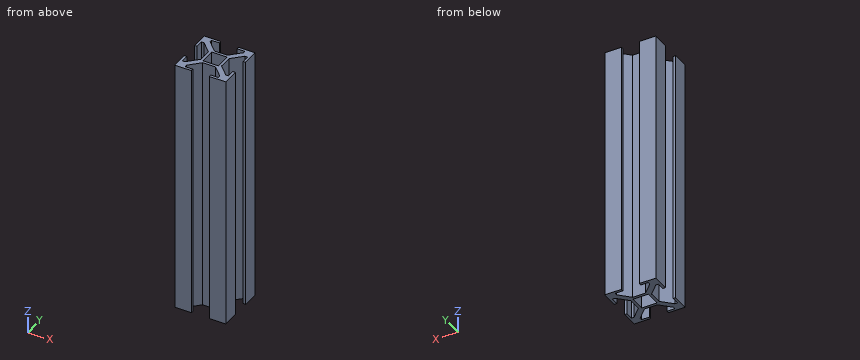
from build123d import *

# Parameters (mm, degrees)
SKETCH_W        = 20
SKETCH_H        = 20
PAD_DEPTH       = 100
SKETCH001_W     = 6
SKETCH001_H     = 6
POCKET_DEPTH    = 100.001
POCKET001_DEPTH = 100.001


with BuildPart() as part:
    # Sketch → Pad (new body)
    with BuildSketch(Plane.XY):
        with Locations((10, 10)):
            Rectangle(SKETCH_W, SKETCH_H)
    extrude(amount=PAD_DEPTH)

    # Sketch001 (on Face6 of Pad) → Pocket (cut, through all)
    with BuildSketch(Plane.XY.offset(100)):
        with Locations((10, 10)):
            Rectangle(SKETCH001_W, SKETCH001_H)
    extrude(amount=-POCKET_DEPTH, mode=Mode.SUBTRACT)

    # Sketch002 (on Face5 of Pocket) → Pocket001 (cut, through all)
    with BuildSketch(Plane.XY.offset(100)):
        Polygon((0, 6.5), (1, 6.5), (1, 3.5), (2, 3.5), (6, 7.5), (6, 12.5), (2, 16.5), (1, 16.5), (1, 13.5), (0, 13.5), align=None)
        Polygon((6.5, 0), (6.5, 1), (3.5, 1), (3.5, 2), (7.5, 6), (12.5, 6), (16.5, 2), (16.5, 1), (13.5, 1), (13.5, 0), align=None)
        Polygon((20, 6.5), (19, 6.5), (19, 3.5), (18, 3.5), (14, 7.5), (14, 12.5), (18, 16.5), (19, 16.5), (19, 13.5), (20, 13.5), align=None)
        Polygon((6.5, 20), (6.5, 19), (3.5, 19), (3.5, 18), (7.5, 14), (12.5, 14), (16.5, 18), (16.5, 19), (13.5, 19), (13.5, 20), align=None)
    extrude(amount=-POCKET001_DEPTH, mode=Mode.SUBTRACT)


solid = part.part
Can you work these out from the model? Positions are in its coordinate system, mm. Give positions to 0.01 mm unless a question says otherwise; leave off trailing zeros. Loops run counter-clockwise (first coordinate to the right, second up) from the corner with the lowest first, then second, coordinate; pieces in that order, holes last. Notation, with made-up numbers: M -17,-8.5 L -7,-8.5 A12 cw -7,-2.5 Z; hole C 26.5,-6 d4. An arc over 180 degrees is marked long. One line per item, written item: value. Start each with the question number.
1) If we section it at A-A, the plane y = 10.5: Write out the boundary of the cut face in (x, z).
2) I'm going to push flat-ended pins straight in: pin 1 (4 mm diameter, centred on y = 9, z = 58.5, fed in from -X); pin 2 (2 mm diameter, centred on x = 16.5, y = 11.5, fed in from +Z); pin 3 (3 mm diameter, centred on y = 10, z = 53, fed in from -X). Where does each tip first touch, or does it pass through?
3) If I drill on line 1 (X direction, y = 15, z = 13.5); line 2 (X direction, y = 18, z = 91.5), over which ranges is the centre line in solid material (lowest first)? Write a range as [from, to].
Completed:
1. outline: M 6,0 L 7,0 L 7,100 L 6,100 Z; M 13,0 L 14,0 L 14,100 L 13,100 Z
2. pin 1: stops at x = 5.5
2. pin 2: passes through
2. pin 3: stops at x = 6
3. line 1: x = [0, 1], [3.5, 6.5], [13.5, 16.5], [19, 20]
3. line 2: x = [0, 3.5], [16.5, 20]
